The model under review builds one solid part; all positions refer to its coordinate system, in mm. Coordinates: 2 decimals unless noted, no trailing zeros. Order: outer loops, then holes, each group sorted by start corner. A loop starts at its lowest first (then second) coordinate and runs counter-clockwise, first axis right, second up. Notation, with made-up numbers: M 68,88.5 L 108,88.5 A32 cw 108,124.5 Z; hole C 77.25,64.25 d1. An arc over 180 degrees is marked long. Answer in a Markdown table with one row per item.
from build123d import *

# Parameters (mm, degrees)
SKETCH_1_W             = 140
SKETCH_1_H             = 200
SKETCH_1_R             = 1.5
EXTRUDE_1_DEPTH        = 4
SKETCH_2_W             = 20
SKETCH_2_H             = 20
EXTRUDE_2_DEPTH        = 4
FILLET_1_R             = 3
FILLET_1_OF_MIRROR_1_R = 3
SKETCH_3_W             = 8
SKETCH_3_H             = 30
SKETCH_3_R             = 1.75
EXTRUDE_3_DEPTH        = 4
FILLET_2_R             = 3
FILLET_2_OF_MIRROR_2_R = 3
FILLET_3_R             = 5
EXTRUDE_4_DEPTH        = 4
SKETCH_5_W             = 8
SKETCH_5_H             = 8
SKETCH_5_R             = 2
EXTRUDE_5_DEPTH        = 4
SKETCH_6_W             = 20
SKETCH_6_H             = 13.1
CUT_EXTRUDE_1_DEPTH    = 10


with BuildPart() as part:
    # 草图1 → 凸台-拉伸1 (new body)
    with BuildSketch(Plane.XY):
        Rectangle(SKETCH_1_W, SKETCH_1_H)
        with Locations((-65, 40)):
            Circle(SKETCH_1_R, mode=Mode.SUBTRACT)
        with Locations(Location((-65, -40, 0), (0, 0, 180))):
            Circle(SKETCH_1_R, mode=Mode.SUBTRACT)
        with Locations((65, -40)):
            Circle(SKETCH_1_R, mode=Mode.SUBTRACT)
        with Locations(Location((65, 40, 0), (0, 0, 180))):
            Circle(SKETCH_1_R, mode=Mode.SUBTRACT)
    extrude(amount=EXTRUDE_1_DEPTH)

    # 草图2 → 凸台-拉伸2 (add)
    with BuildSketch(Plane.XY.offset(4)):
        with Locations((80, 90)):
            Rectangle(SKETCH_2_W, SKETCH_2_H)
    extrude_2 = extrude(amount=-EXTRUDE_2_DEPTH)

    # 圆角1
    fillet_1_edges = [part.edges().sort_by_distance(p)[0] for p in [
        (90, 100, 2),
        (90, 80, 2),
    ]]
    fillet(fillet_1_edges, radius=FILLET_1_R)

    # 镜向1: 凸台-拉伸2 across plane
    add(extrude_2.mirror(Plane(origin=(0, 0, 0), x_dir=(0, 0, 1), z_dir=(1, 0, 0))))

    # 圆角1 of 镜向1
    fillet_1_of_mirror_1_edges = [part.edges().sort_by_distance(p)[0] for p in [
        (-90, 100, 2),
        (-90, 80, 2),
    ]]
    fillet(fillet_1_of_mirror_1_edges, radius=FILLET_1_OF_MIRROR_1_R)

    # 草图3 → 凸台-拉伸3 (add)
    with BuildSketch(Plane.XY.offset(4)):
        with Locations((-66, 115)):
            Rectangle(SKETCH_3_W, SKETCH_3_H)
        with Locations((-66, 126)):
            Circle(SKETCH_3_R, mode=Mode.SUBTRACT)
    extrude_3 = extrude(amount=-EXTRUDE_3_DEPTH)

    # 圆角2
    fillet_2_edges = [part.edges().sort_by_distance(p)[0] for p in [
        (-70, 100, 2),
        (-62, 100, 2),
    ]]
    fillet(fillet_2_edges, radius=FILLET_2_R)

    # 镜向2: 凸台-拉伸3 across plane
    add(extrude_3.mirror(Plane(origin=(0, 0, 0), x_dir=(0, 0, 1), z_dir=(1, 0, 0))))

    # 圆角2 of 镜向2
    fillet_2_of_mirror_2_edges = [part.edges().sort_by_distance(p)[0] for p in [
        (70, 100, 2),
        (62, 100, 2),
    ]]
    fillet(fillet_2_of_mirror_2_edges, radius=FILLET_2_OF_MIRROR_2_R)

    # 圆角3
    fillet_3_edges = [part.edges().sort_by_distance(p)[0] for p in [
        (-70, -100, 2),
        (70, -100, 2),
    ]]
    fillet(fillet_3_edges, radius=FILLET_3_R)

    # 草图4 → 凸台-拉伸4 (add)
    with BuildSketch(Plane(origin=(0, 0, 0), x_dir=(-1, 0, 0), z_dir=(0, 0, -1))):
        with BuildLine():
            add(Edge.make_bspline(
                [(-33.786379938, 100), (-33.384771108, 111.24314249), (-38.944167614, 121.897129031), (-48.25387443, 128.002822688)],
                knots=[0, 0, 0, 0, 0.66194058, 0.66194058, 0.66194058, 0.66194058], degree=3))
            Line((-33.786379938, 100), (0, 100))
            ThreePointArc((0, 100), (-9.331566745, 102.310402433), (-16.507166038, 108.707813791))
            ThreePointArc((-16.507166038, 108.707813791), (-29.663945789, 122.555538901), (-46.506293223, 131.566403293))
            ThreePointArc((-46.506293223, 131.566403293), (-48.952735362, 130.555841868), (-48.25387443, 128.002822688))
        make_face()
        with BuildLine():
            ThreePointArc((16.507166038, 108.707813791), (9.331566745, 102.310402433), (0, 100))
            Line((0, 100), (33.786379938, 100))
            add(Edge.make_bspline(
                [(33.786379938, 100), (33.384771108, 111.24314249), (38.944167614, 121.897129031), (48.25387443, 128.002822688)],
                knots=[0, 0, 0, 0, 0.66194058, 0.66194058, 0.66194058, 0.66194058], degree=3))
            ThreePointArc((48.25387443, 128.002822688), (48.952735362, 130.555841868), (46.506293223, 131.566403293))
            ThreePointArc((46.506293223, 131.566403293), (29.663945789, 122.555538901), (16.507166038, 108.707813791))
        make_face()
    extrude(amount=-EXTRUDE_4_DEPTH)

    # 草图5 → 凸台-拉伸5 (add)
    # profile 1 of 2: a face of its own
    with BuildSketch(Plane.XY.offset(4)):
        with Locations((-74, 0)):
            Rectangle(SKETCH_5_W, SKETCH_5_H)
        with Locations((-74, 0)):
            Circle(SKETCH_5_R, mode=Mode.SUBTRACT)
    # profile 2 of 2: a face of its own
    with BuildSketch(Plane.XY.offset(4)):
        with Locations((74, 0)):
            Rectangle(SKETCH_5_W, SKETCH_5_H)
        with Locations(Location((74, 0, 0), (0, 0, 180))):
            Circle(SKETCH_5_R, mode=Mode.SUBTRACT)
    extrude(amount=-EXTRUDE_5_DEPTH)

    # 草图6 → 切除-拉伸1 (cut)
    with BuildSketch(Plane.XY.offset(4)):
        with Locations((-15, 83.45)):
            Rectangle(SKETCH_6_W, SKETCH_6_H)
        with Locations((15, 83.45)):
            Rectangle(SKETCH_6_W, SKETCH_6_H)
        with BuildLine():
            Line((-23.45, 74.95), (-6.55, 74.95))
            ThreePointArc((-6.55, 74.95), (-5, 73.4), (-6.55, 71.85))
            Line((-6.55, 71.85), (-23.45, 71.85))
            ThreePointArc((-23.45, 71.85), (-25, 73.4), (-23.45, 74.95))
        make_face()
        with BuildLine():
            Line((23.45, 71.85), (6.55, 71.85))
            ThreePointArc((6.55, 71.85), (5, 73.4), (6.55, 74.95))
            Line((6.55, 74.95), (23.45, 74.95))
            ThreePointArc((23.45, 74.95), (25, 73.4), (23.45, 71.85))
        make_face()
    extrude(amount=-CUT_EXTRUDE_1_DEPTH, mode=Mode.SUBTRACT)


solid = part.part
(1) Insertion check: P1, Ø2, axis at x = -75, z = 3, coming from the +Y side; P2, Ø1.5, axis at y = 2, z = 3.5, coming from the +X side; P3, Ø2, axis at y = 115, z = 1.5, coming from the -X side. Each pin has a flat end and moves straight along its axis. Give the tip position at first contact, or say it passes through.
Report:
| item | result |
|---|---|
| P1 | y = 100 |
| P2 | x = 78 |
| P3 | x = -70 |
(2) The part is to be moulded in two halves that separate along X. For faces 1 (the cylindrical face through (-29.88, 122.72, 1.97)), 2 (the cylindrical face through (29.45, 122.39, 1.97)), 3 (the cylindrical face through (-69, -98, 2)), 4 (the flat face through (-1, 17, 0)), say which applies: +X half, -X half, draft (parallel to the pull), parting line (faces both ways), or undercut.
Report:
| item | result |
|---|---|
| face 1 | undercut |
| face 2 | undercut |
| face 3 | -X half |
| face 4 | draft |
(3) Take a section at C-C (x = 29). Write out the cut boundary in (y, z), then the cut area to 3 significant figures.
Report:
| item | result |
|---|---|
| outline | M -100,0 L 122.04,0 L 122.04,4 L -100,4 Z |
| area | 888 mm^2 |
(4) To check wall thickness, follow line 1 (Y direction, x = -74, z = 2.75); line 2 (Y direction, x = -65, z = 1.95); line 3 (Y direction, x = -15.5, z = 1.6). State the ranges of each line that lie inside material, in increasing order. Write a range as [from, to].
Report:
| item | result |
|---|---|
| line 1 | [-4, -2], [2, 4], [80, 100] |
| line 2 | [-100, -41.5], [-38.5, 38.5], [41.5, 124.56], [127.44, 130] |
| line 3 | [-100, 71.85], [74.95, 76.9], [90, 107.36] |
(5) Take a section at A-A (y = 111.5). State how many separate pieces and enclosed holes the cut face has, then the cut area to 3 significant figures.
Report:
| item | result |
|---|---|
| separate pieces | 4 |
| enclosed holes | 0 |
| area | 200 mm^2 |
